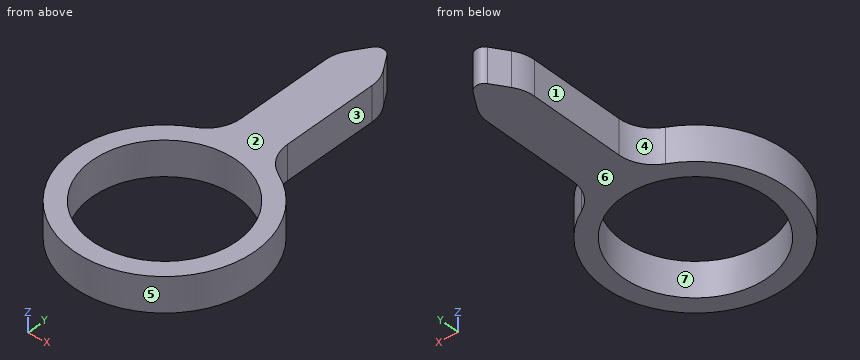
```python
from build123d import *

# Parameters (mm, degrees)
SKETCH1_R           = 3.302
BOSS_EXTRUDE1_DEPTH = 1.5875
FILLET1_R           = 1.5875
FILLET2_R           = 0.396875
FILLET3_R           = 1.5875


with BuildPart() as part:
    # Sketch1 → Boss-Extrude1 (new body)
    with BuildSketch(Plane.XY):
        with BuildLine():
            Line((1.05664, 3.989958416), (1.05664, 9.8425))
            Line((1.05664, 9.8425), (0, 11.43))
            Line((0, 11.43), (-1.05664, 9.8425))
            Line((-1.05664, 9.8425), (-1.05664, 3.989958416))
            ThreePointArc((-1.05664, 3.989958416), (0, -4.1275), (1.05664, 3.989958416))
        make_face()
        Circle(SKETCH1_R, mode=Mode.SUBTRACT)
    extrude(amount=BOSS_EXTRUDE1_DEPTH)

    # Fillet1
    fillet1_edges = [part.edges().sort_by_distance(p)[0] for p in [
        (1.05664, 9.8425, 0.79375),
        (-1.05664, 9.8425, 0.79375),
    ]]
    fillet(fillet1_edges, radius=FILLET1_R)

    # Fillet2
    fillet2_edges = [part.edges().sort_by_distance(p)[0] for p in [
        (0, 11.43, 0.79375),
    ]]
    fillet(fillet2_edges, radius=FILLET2_R)

    # Fillet3
    fillet3_edges = [part.edges().sort_by_distance(p)[0] for p in [
        (1.05664, 3.989958416, 0.79375),
        (-1.05664, 3.989958416, 0.79375),
    ]]
    fillet(fillet3_edges, radius=FILLET3_R)


solid = part.part
```
Here's how the part is built. I have some questions about the finished solid (model axes, mm). Face numbers are marked on the shaded views. A direction names the side the tool comes from. Coordinates: 2 decimals unless noted, no trailing zeros. Write each loop counter-clockwise with the first axis right and the second up, starting at its lowest first coordinate (ties: lowest second). Pieces come first, ordered by that corner, then holes. Notation, with made-up numbers: (-17.5, -28) -> (23.5, -28) arc R7 cw to (23.5, -24) -> close; hole circle Ø2 at (-8.75, 28.5). An arc over 180 degrees is marked (long way). Use a Markdown table: item, result. Add a question column.
(1) If we section it at C-C, the plane z = 0.2: Write out the boundary of the cut face in (x, y) (1 decimal).
(2) We'd pull the mould along Y, two halves only. Please class the marked faces 4, 5, 6 and 7: +Y half, -Y half, draft (parallel to the pull), parting line (faces both ways), or undercut.
(3) For the marked faces 1, 2 and 3, which set-ups out of +Z, -Z, +X, -X, +Y, -Y let a thin tool reach every point of the face, with its end or its side?
(4) I'm going to push a flat-ended pin straight in: P1, Ø0.8, axis at y = 8, z = 0.5, coming from the +X side. Where does the tip first touch, or does it pass through?
(5) If we section it at A-A, the plane y = 0: Write out the boundary of the cut face in (x, z), and give its area (3 significant figures).
(6) Please list where these lines run through material, in increasing order: line 1 (X direction, y = 5.5, z = 0.15); line 2 (Y direction, x = -0.5, z = 1.55); line 3 (Y direction, x = -2, z = 1.5).
(7) If we section it at B-B, the plane x = 0: Write out the boundary of the cut face in (y, z), and give its area (3 significant figures).
(8) If we section it at D-D, the plane y = 7.5: Write out the boundary of the cut face in (x, z), and give its area (3 significant figures).
Outcome:
| question | item | result |
|---|---|---|
| 1 | outline | (-1.9, 3.7) arc R4.1 ccw (long way) to (1.9, 3.7) arc R1.6 cw to (1.1, 5.1) -> (1.1, 9.4) arc R1.6 ccw to (0.8, 10.2) -> (0.3, 10.9) arc R0.4 ccw to (-0.3, 10.9) -> (-0.8, 10.2) arc R1.6 ccw to (-1.1, 9.4) -> (-1.1, 5.1) arc R1.6 cw to start; hole circle Ø6.6 at (0, 0) |
| 2 | face 4 | +Y half |
| 2 | face 5 | parting line |
| 2 | face 6 | draft |
| 2 | face 7 | undercut |
| 3 | face 1 | +Z, -Z, -X, +Y |
| 3 | face 2 | +Z, +X, -X, +Y, -Y |
| 3 | face 3 | +Z, -Z, +X, +Y |
| 4 | P1 | stops at x = 1.06 |
| 5 | outline | (-4.13, 0) -> (-3.3, 0) -> (-3.3, 1.59) -> (-4.13, 1.59) -> close; (3.3, 0) -> (4.13, 0) -> (4.13, 1.59) -> (3.3, 1.59) -> close |
| 5 | area | 2.62 mm^2 |
| 6 | line 1 | x = -1.06 to 1.06 |
| 6 | line 2 | y = -4.1 to -3.26, 3.26 to 10.68 |
| 6 | line 3 | y = -3.61 to -2.63, 2.63 to 3.61 |
| 7 | outline | (-4.13, 0) -> (-3.3, 0) -> (-3.3, 1.59) -> (-4.13, 1.59) -> close; (3.3, 0) -> (11.11, 0) -> (11.11, 1.59) -> (3.3, 1.59) -> close |
| 7 | area | 13.7 mm^2 |
| 8 | outline | (-1.06, 0) -> (1.06, 0) -> (1.06, 1.59) -> (-1.06, 1.59) -> close |
| 8 | area | 3.35 mm^2 |
